For this review, take the finished solid that the model builds, in its own axes (mm). Face numbers are marked on the shaded views. A direction names the side the tool comes from. Give positions to 0.01 mm unless a question says otherwise; leave off trailing zeros. Loops run counter-clockwise (first coordinate to the right, second up) from the corner with the lowest first, then second, coordinate; pieces in that order, holes last. Notation, with made-up numbers: (78, 48.25) - (99, 48.25) arc R32 ccw to (99, 81.25) - close; hole circle Ø9 at (-13, -20). An arc over 180 degrees is marked (long way). Answer in a Markdown table with one row per item.
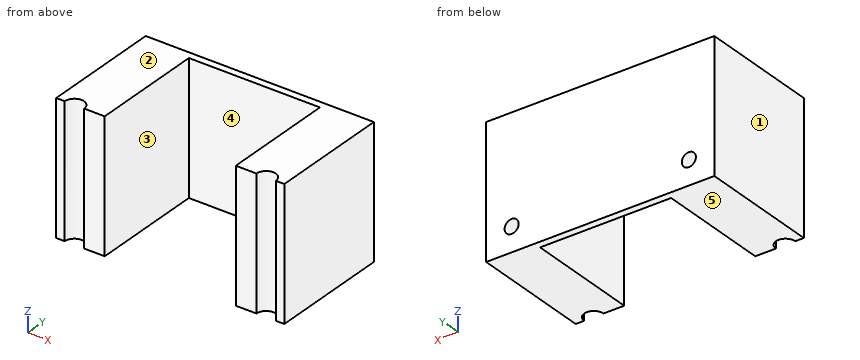
```python
from build123d import *

# Parameters (mm, degrees)
PAD_DEPTH       = 27
SKETCH001_R     = 2
POCKET_DEPTH    = 27.001
SKETCH002_R     = 1.45
POCKET001_DEPTH = 10


with BuildPart() as part:
    # Sketch → Pad (new body)
    with BuildSketch(Plane.XY):
        Polygon((13.5, 0), (13.5, 23.5), (-13.5, 23.5), (-13.5, 0), (-23.5, 0), (-23.5, 25), (23.5, 25), (23.5, 0), align=None)
    extrude(amount=PAD_DEPTH)

    # Sketch001 → Pocket (cut, through all)
    with BuildSketch(Plane.XY):
        with Locations((-19.75, 0)):
            Circle(SKETCH001_R)
        with Locations((19.75, 0)):
            Circle(SKETCH001_R)
    extrude(amount=POCKET_DEPTH, mode=Mode.SUBTRACT)

    # Sketch002 (on DatumPlane) → Pocket001 (cut)
    with BuildSketch(Plane.XZ.offset(-25)):
        with Locations((-18.25, 5)):
            Circle(SKETCH002_R)
        with Locations((18.25, 5)):
            Circle(SKETCH002_R)
    extrude(amount=POCKET001_DEPTH, mode=Mode.SUBTRACT)


solid = part.part
```
1. For the marked faces 4 and 5, list the 3-axis set-ups (+Z, -Z, +X, -X, +Y, -Y) from which the entire face can be reached by the end or side of a thin tool; tool diameter is ignored.
Values:
| item | result |
|---|---|
| face 4 | +Z, -Z, -Y |
| face 5 | -Z, +X, -X, +Y, -Y |
2. We need section D-D, the plane x = -18.25. Give the boundary of the cut face in (y, z), and give its area (3 significant figures).
Values:
| item | result |
|---|---|
| outline | (1.32, 0) - (25, 0) - (25, 3.55) - (15, 3.55) - (15, 6.45) - (25, 6.45) - (25, 27) - (1.32, 27) - close |
| area | 610 mm^2 |
3. We need section C-C, the plane z = 5. Give the boundary of the cut face in (x, y), and give its area (3 significant figures).
Values:
| item | result |
|---|---|
| outline | (-23.5, 0) - (-21.75, 0) arc R2 cw to (-17.75, 0) - (-13.5, 0) - (-13.5, 23.5) - (13.5, 23.5) - (13.5, 0) - (17.75, 0) arc R2 cw to (21.75, 0) - (23.5, 0) - (23.5, 25) - (19.7, 25) - (19.7, 15) - (16.8, 15) - (16.8, 25) - (-16.8, 25) - (-16.8, 15) - (-19.7, 15) - (-19.7, 25) - (-23.5, 25) - close |
| area | 470 mm^2 |
4. We need section A-A, the plane y = 23. Give the boundary of the cut face in (x, z), and give its area (3 significant figures).
Values:
| item | result |
|---|---|
| outline | (-23.5, 0) - (-13.5, 0) - (-13.5, 27) - (-23.5, 27) - close; (13.5, 0) - (23.5, 0) - (23.5, 27) - (13.5, 27) - close; hole circle Ø2.9 at (-18.25, 5); hole circle Ø2.9 at (18.25, 5) |
| area | 527 mm^2 |
5. Clearance check with flat-ended pins moving along their axes: pin 1 (2 mm diameter, centred on x = 2.5, z = 10.5, fed in from -Y); pin 2 (0.9 mm diameter, centred on x = 18, z = 4.5, fed in from +Y). State where each tip first meets the part, or that it passes through.
Values:
| item | result |
|---|---|
| pin 1 | stops at y = 23.5 |
| pin 2 | stops at y = 15 |
6. We need section B-B, the plane y = 4.5. Give the boundary of the cut face in (x, z), and give its area (3 significant figures).
Values:
| item | result |
|---|---|
| outline | (-23.5, 0) - (-13.5, 0) - (-13.5, 27) - (-23.5, 27) - close; (13.5, 0) - (23.5, 0) - (23.5, 27) - (13.5, 27) - close |
| area | 540 mm^2 |
7. Wall thickness on line 1 (Z direction, x = -18.25, y = 20.75); line 2 (X direction, y = 9, z = 3.25); line 3 (Y direction, x = 13, z = 26): over which ranges is each line inside the solid? List them lowest first. Write a range as [from, to].
Values:
| item | result |
|---|---|
| line 1 | z = [0, 3.55], [6.45, 27] |
| line 2 | x = [-23.5, -13.5], [13.5, 23.5] |
| line 3 | y = [23.5, 25] |
8. Mouldability with a two-part tool opening along X and no side actions: class the marked faces 1, 2 and 3 as released by +X, released by -X, zero draft, split by the parting line, or undercut.
Values:
| item | result |
|---|---|
| face 1 | released by -X |
| face 2 | zero draft |
| face 3 | undercut |
